Autodesk Inventor part; units mm, degrees
ref_plane "actu_a_right_XY" through (-0.0508, 0, 3.2385) normal (0, 0, -1) x (1, 0, 0)
ref_plane "actu_a_right_YZ" through (-0.0508, 0, 3.2385) normal (1, 0, 0) x (0, -1, 0)
ref_plane "actu_a_right_ZX" through (-0.0508, 0, 3.2385) normal (0, -1, 0) x (0, 0, -1)
sketch "Sketch_1" plane through (0, 0, 0) normal (0, 0, 1) x (1, 0, 0)
  line L0 (-4.4958, -2.3876) -> (-4.3434, -2.54)
  line L1 (-4.3434, -2.54) -> (4.3434, -2.54)
  line L2 (4.3434, -2.54) -> (4.4958, -2.3876)
  line L3 (4.4958, -2.3876) -> (4.4958, 2.3876)
  line L4 (4.4958, 2.3876) -> (4.3434, 2.54)
  line L5 (4.3434, 2.54) -> (-4.3434, 2.54)
  line L6 (-4.3434, 2.54) -> (-4.4958, 2.3876)
  line L7 (-4.4958, 2.3876) -> (-4.4958, -2.3876)
extrude "Extrusion1" add sketch "Sketch_1" along normal blind 4.1529
sketch "Sketch_5" plane through (0, 0, 4.1529) normal (0, 0, 1) x (1, 0, 0)
  line L0 (-2.4384, 1.1938) -> (-2.4384, -1.1938)
  line L1 (-2.4384, -1.1938) -> (2.4384, -1.1938)
  line L2 (2.4384, -1.1938) -> (2.4384, 1.1938)
  line L3 (2.4384, 1.1938) -> (-2.4384, 1.1938)
extrude "Extrusion2" cut sketch "Sketch_5" against normal blind 0.9144
sketch "Sketch_4" plane through (4.4958, 0, 0) normal (1, 0, 0) x (0, 0, -1)
  line L0 (-2.54, 1.27) -> (-2.54, -1.27)
  line L1 (-2.54, -1.27) -> (-1.9304, -1.27)
  line L2 (-1.9304, -1.27) -> (-1.9304, 1.27)
  line L3 (-1.9304, 1.27) -> (-2.54, 1.27)
extrude "Extrusion3" cut sketch "Sketch_4" against normal blind 0.254
sketch "Sketch_6" plane through (-4.4958, 0, 0) normal (1, 0, 0) x (0, 0, -1)
  line L0 (-2.54, 1.27) -> (-2.54, -1.27)
  line L1 (-2.54, -1.27) -> (-1.9304, -1.27)
  line L2 (-1.9304, -1.27) -> (-1.9304, 1.27)
  line L3 (-1.9304, 1.27) -> (-2.54, 1.27)
extrude "Extrusion4" cut sketch "Sketch_6" along normal blind 0.254
sketch "Sketch_2" plane through (0, 0, 0) normal (0, 0, 1) x (1, 0, 0)
  line L0 (-3.8862, 2.54) -> (-3.8862, -2.54)
  line L1 (-3.8862, -2.54) -> (3.8862, -2.54)
  line L2 (3.8862, -2.54) -> (3.8862, 2.54)
  line L3 (3.8862, 2.54) -> (-3.8862, 2.54)
extrude "Extrusion5" cut sketch "Sketch_2" along normal blind 0.6096
ref_plane "actu_a_right_XY" through (-0.0508, 0, 3.2385) normal (0, 0, -1) x (1, 0, 0)
ref_plane "actu_a_right_YZ" through (-0.0508, 0, 3.2385) normal (1, 0, 0) x (0, -1, 0)
ref_plane "actu_a_right_ZX" through (-0.0508, 0, 3.2385) normal (0, -1, 0) x (0, 0, -1)
ref_plane "body12_right_XY" through (0, 0, 0.6096) normal (0, 0, 1) x (1, 0, 0)
ref_plane "body12_right_YZ" through (0, 0, 0.6096) normal (1, 0, 0) x (0, 1, 0)
ref_plane "body12_right_ZX" through (0, 0, 0.6096) normal (0, 1, 0) x (0, 0, 1)
properties part number "AS11CHright1"
CAD build for the part. Positions are in the model's coordinates, mm. A direction names the side the tool comes from. Round coordinates to 2 decimals unless told otherwise and drop trailing zeros. Order: outer loops, then holes, each group sorted by start corner. A loop starts at its lowest first (then second) coordinate and runs counter-clockwise, first axis right, second up. Notation, with made-up numbers: (21.5, -18.5) -> (57.5, -18.5) arc R30 ccw to (57.5, 16.5) -> close; hole circle Ø4 at (10.25, 37). An arc over 180 degrees is marked (long way). Write each question's results on one line, items separated by ' | '.
1. Cut at D-D (z = 3.35). Give the cut face in (x, y), plus the area to 3 significant figures.
Findings below:
outline: (-4.5, -2.39) -> (-4.34, -2.54) -> (4.34, -2.54) -> (4.5, -2.39) -> (4.5, 2.39) -> (4.34, 2.54) -> (-4.34, 2.54) -> (-4.5, 2.39) -> close; hole (-2.44, -1.19) -> (2.44, -1.19) -> (2.44, 1.19) -> (-2.44, 1.19) -> close | area: 34.0 mm²
2. Cut at B-B (y = -0.05). Give the cut face in (x, z).
Findings below:
outline: (-4.5, 0) -> (-3.89, 0) -> (-3.89, 0.61) -> (3.89, 0.61) -> (3.89, 0) -> (4.5, 0) -> (4.5, 1.93) -> (4.24, 1.93) -> (4.24, 2.54) -> (4.5, 2.54) -> (4.5, 4.15) -> (2.44, 4.15) -> (2.44, 3.24) -> (-2.44, 3.24) -> (-2.44, 4.15) -> (-4.5, 4.15) -> (-4.5, 2.54) -> (-4.24, 2.54) -> (-4.24, 1.93) -> (-4.5, 1.93) -> close
3. Wall check: line 1 along X through (y, z) = (-0.8, 3.4); line 2 along Y through (x, z) = (1.75, 3.4); line 3 along Z through (x, y) = (0.25, -0.2). Give the ranges that are in metal, low to high. Write a range as [from, to].
Findings below:
line 1: x = [-4.5, -2.44], [2.44, 4.5] | line 2: y = [-2.54, -1.19], [1.19, 2.54] | line 3: z = [0.61, 3.24]
4. 3-axis set-ups, long thin cutter, end or side, ignore diameter. For faces 1 (the face through (0, 0, 3.238)), 2 (the face through (0, 0, 0.61)), 3 (the face through (0, -2.54, 2)): which of +Z, -Z, +X, -X, +Y, -Y reach the whole face in a straight line?
Findings below:
face 1: +Z | face 2: -Z, +Y, -Y | face 3: +Z, -Z, +X, -X, -Y
5. Flat gauge pins, fed straight in: P1, Ø2.5, axis at x = -1, y = 0.5, coming from the -Z side; P2, Ø1.9, axis at x = 0, y = 0.5, coming from the +Z side. Where does each tip first touch, or does it go through?
Findings below:
P1: stops at z = 0.61 | P2: stops at z = 4.15
6. Cut at A-A (z = 0.35). Give the cut face in (x, y).
Findings below:
outline: (-4.5, -2.39) -> (-4.34, -2.54) -> (-3.89, -2.54) -> (-3.89, 2.54) -> (-4.34, 2.54) -> (-4.5, 2.39) -> close; (3.89, -2.54) -> (4.34, -2.54) -> (4.5, -2.39) -> (4.5, 2.39) -> (4.34, 2.54) -> (3.89, 2.54) -> close
7. Cut at C-C (x = 2.25). Give the cut face in (y, z).
Findings below:
outline: (-2.54, 0.61) -> (2.54, 0.61) -> (2.54, 4.15) -> (1.19, 4.15) -> (1.19, 3.24) -> (-1.19, 3.24) -> (-1.19, 4.15) -> (-2.54, 4.15) -> close
8. Pull direction X, two halves, no side cores. Call faces 4 (the face through (2.438, 0, 4)), 5 (the face through (-4.496, 0, 1.6)), 6 (the face through (0, 2.54, 2)): pulls with the +X half, pulls with the -X half, needs draft (parallel to the pull), parting line crosses it, or undercut.
Findings below:
face 4: undercut | face 5: pulls with the -X half | face 6: needs draft
